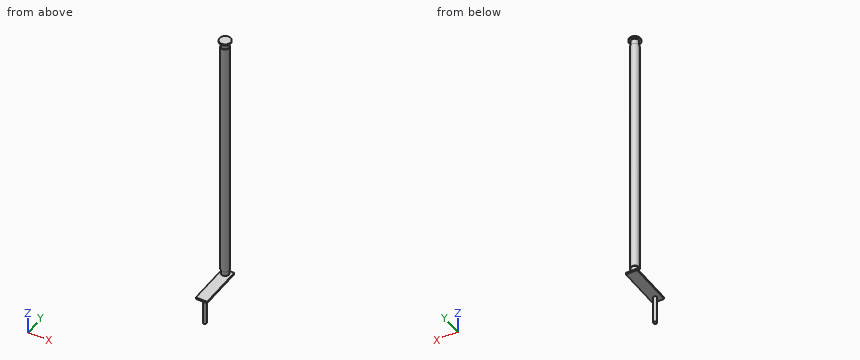
Autodesk Inventor part; units mm, degrees
ref_plane "YZ Plane" through (0, 0, 0) normal (1, 0, 0) x (0, 1, 0)
ref_plane "XZ Plane" through (0, 0, 0) normal (0, 1, 0) x (-1, 0, 0)
ref_plane "XY Plane" through (0, 0, 0) normal (0, 0, 1) x (1, 0, 0)
sketch "Sketch1" plane through (0, 0, 0) normal (0, 0, 1) x (1, 0, 0)
  circle A0 centre (0, 0) radius 25
  dimension "d0" = 50
extrude "Extrusion1" add sketch "Sketch1" along normal blind 10
sketch "Sketch2" plane through (0, 0, 10) normal (0, 0, 1) x (1, 0, 0)
  circle A0 centre (0, 0) radius 6.5
  dimension "d3" = 13
extrude "Extrusion2" add sketch "Sketch2" along normal blind 10
fillet "Fillet1" radius 1 1 edges at (-6.5, 0, 10)
sketch "Sketch4" plane through (0, 0, 0) normal (0, 0, -1) x (-1, 0, 0)
  arc A0 (19.3649, 5) -> (5, 19.3649) centre (0, 0) ccw
  line L0 (2.5, 17.4284) -> (2.5, 9.4868)
  line L1 (9.4868, 2.5) -> (17.4284, 2.5)
  arc A1 (5, 19.3649) -> (2.5, 17.4284) centre (4.5, 17.4284) ccw
  arc A2 (17.4284, 2.5) -> (19.3649, 5) centre (17.4284, 4.5) ccw
  arc A3 (2.5, 8.3666) -> (2.5153, 8.1193) centre (4.5, 8.3666) ccw
  arc A4 (8.1193, 2.5153) -> (8.3666, 2.5) centre (8.3666, 4.5) ccw
  arc A5 (7.6798, 3.6429) -> (3.6429, 7.6798) centre (0, 0) ccw
  arc A6 (2.5, 9.4868) -> (3.6429, 7.6798) centre (4.5, 9.4868) ccw
  arc A7 (7.6798, 3.6429) -> (9.4868, 2.5) centre (9.4868, 4.5) ccw
  point P0 (2.5, 19.8431)
  point P1 (19.8431, 2.5)
  point P2 (2.5, 7.0711)
  point P3 (7.0711, 2.5)
extrude "Extrusion3" cut sketch "Sketch4" against normal blind 10
pattern_circular "Circular Pattern1" count 4 over 360 about axis through (0, 0, 11) along (0, 0, -1) of "Extrusion3"
sketch "Sketch7" plane through (0, 0, 20) normal (0, 0, 1) x (1, 0, 0)
  circle A0 centre (0, 0) radius 7.5
  dimension "d38" = 15
extrude "Extrusion5" add sketch "Sketch7" along normal blind 440
sketch "Sketch8" plane through (0, 0, 460) normal (0, 0, 1) x (1, 0, 0)
  circle A0 centre (0, 0) radius 6.5
  dimension "d41" = 13
extrude "Extrusion6" add sketch "Sketch8" along normal blind 10
sketch "Sketch9" plane through (0, 0, 470) normal (0, 0, 1) x (1, 0, 0)
  circle A0 centre (0, 0) radius 10
  dimension "d44" = 20
extrude "Extrusion7" add sketch "Sketch9" along normal blind 2.5
thread "Thread1"
sketch "Sketch10" plane through (0, 0, 0) normal (0, 0, -1) x (-1, 0, 0)
  circle A0 centre (0, 0) radius 25
extrude "Extrusion8" cut sketch "Sketch10" against normal blind 10
sketch "Sketch11" plane through (0, 0, 10) normal (0, 0, -1) x (-1, 0, 0)
  circle A0 centre (0, 0) radius 10
extrude "Extrusion9" cut sketch "Sketch11" against normal blind 1
sketch "Sketch12" plane through (0, 0, 11) normal (0, 0, -1) x (-1, 0, 0)
  circle A0 centre (0, 0) radius 3
  dimension "d53" = 6
extrude "Extrusion10" add sketch "Sketch12" along normal blind 5
sketch "Sketch13" plane through (0, 0, 6) normal (0, 0, -1) x (-1, 0, 0)
  circle A0 centre (0, 0) radius 3
  circle A1 centre (0, 0) radius 3
  line L0 (-10, 10) -> (10, 10)
  line L1 (10, 10) -> (10, -70)
  line L2 (10, -70) -> (-10, -70)
  line L3 (-10, -70) -> (-10, 10)
  dimension "d56" = 80
extrude "Extrusion11" add sketch "Sketch13" against normal blind 3
sketch "Sketch14" plane through (0, 0, 6) normal (0, 0, -1) x (-1, 0, 0)
  line L0 (10, -70) -> (-10, -70)
  circle A0 centre (0, -60) radius 3
  point P0 (0, 0)
  dimension "d60" = 6
extrude "Extrusion12" add sketch "Sketch14" along normal blind 50
properties part number "leadscrew_modified_long" material "Steel, Alloy"
The model under review builds one solid part; all positions refer to its coordinate system, in mm. Round coordinates to 2 decimals unless told otherwise and drop trailing zeros. Loops run counter-clockwise (first coordinate to the right, second up) from the corner with the lowest first, then second, coordinate; pieces in that order, holes last. Notation, with made-up numbers: M 56,-15 L 75,-15 A26 cw 75,1 Z; hole C 13.25,47.25 d3. An arc over 180 degrees is marked long. Put each result on its own line as item: value.
Q1. Consider section B-B, the plane z = 359. Give the boundary of the cut face in (x, y).
Result set:
outline: C 0,0 d15
Q2. For pin 1 (2 mm diameter, centred on x = -0.5, y = -50, fed in from +Z); pin 2 (4 mm diameter, centred on x = 1, y = 0.5, fed in from -Z); pin 3 (3 mm diameter, centred on x = -2, z = 126.5, fed in from +Y), all flat-tipped, find the tip position at first contact; note any pin that passes through.
Result set:
pin 1: stops at z = 9
pin 2: stops at z = 6
pin 3: stops at y = 7.48
Q3. Consider section A-A, the plane x = 0. Give the boundary of the cut face in (y, z), then the cut area to 3 significant figures.
Result set:
outline: M -70,6 L -63,6 L -63,-44 L -57,-44 L -57,6 L 10,6 L 10,9 L 3,9 L 3,11 L 6.5,11 L 6.5,20 L 7.5,20 L 7.5,460 L 6.5,460 L 6.5,470 L 10,470 L 10,472.5 L -10,472.5 L -10,470 L -6.5,470 L -6.5,460 L -7.5,460 L -7.5,20 L -6.5,20 L -6.5,11 L -3,11 L -3,9 L -70,9 Z
area: 7,450 mm²
Q4. Consider section C-C, the plane y = -49. Give the boundary of the cut face in (x, z), then the cut area to 3 significant figures.
Result set:
outline: M -10,6 L 10,6 L 10,9 L -10,9 Z
area: 60.0 mm²
Q5. To check wall thickness, follow L1, parallel to Z at x = 7, y = -4.5; L2, parallel to Z at x = 1.75, y = 4; L3, parallel to Z at x = -8.25, y = -64. State the ranges of each line that lie inside material, in increasing order.
Result set:
L1: z = 6 to 9, 470 to 472.5
L2: z = 6 to 9, 11 to 472.5
L3: z = 6 to 9
